Design review of the part built by this model. Coordinates are the model's own, in mm. Coordinates: 2 decimals unless noted, no trailing zeros. Loops run counter-clockwise (first coordinate to the right, second up) from the corner with the lowest first, then second, coordinate; pieces in that order, holes last. Notation, with made-up numbers: M 61.25,-2.75 L 104.25,-2.75 A14 cw 104.25,19.25 Z; hole C 11,37.5 d9. An arc over 180 degrees is marked long. Write item = value, one per line. Start each with the question number.
from build123d import *

# Parameters (mm, degrees)
ESQUISSE1_W        = 35
ESQUISSE1_H        = 23
ESQUISSE1_R        = 3.5
ESQUISSE1_R_2      = 1
ESQUISSE1_R_3      = 1.5
BOSS_EXTRU_1_DEPTH = 6


with BuildPart() as part:
    # Esquisse1 → Boss.-Extru.1 (new body)
    with BuildSketch(Plane.XY):
        Rectangle(ESQUISSE1_W, ESQUISSE1_H)
        Circle(ESQUISSE1_R, mode=Mode.SUBTRACT)
        with Locations((0, 8)):
            Circle(ESQUISSE1_R_2, mode=Mode.SUBTRACT)
        with Locations((8, 0)):
            Circle(ESQUISSE1_R_2, mode=Mode.SUBTRACT)
        with Locations((0, -8)):
            Circle(ESQUISSE1_R_2, mode=Mode.SUBTRACT)
        with Locations((-8, 0)):
            Circle(ESQUISSE1_R_2, mode=Mode.SUBTRACT)
        with Locations((-14.5, 5.75)):
            Circle(ESQUISSE1_R_3, mode=Mode.SUBTRACT)
        with Locations(Location((-14.5, -5.75, 0), (0, 0, 180))):
            Circle(ESQUISSE1_R_3, mode=Mode.SUBTRACT)
        with Locations((14.5, -5.75)):
            Circle(ESQUISSE1_R_3, mode=Mode.SUBTRACT)
        with Locations(Location((14.5, 5.75, 0), (0, 0, 180))):
            Circle(ESQUISSE1_R_3, mode=Mode.SUBTRACT)
    extrude(amount=BOSS_EXTRU_1_DEPTH)


solid = part.part
Q1. Add section D-D on z = 4.95. Give the number of separate pieces and of enclosed holes in the cut face, plus the area to 3 significant figures.
Q2. Add section C-C on y = 0. State the section outline as (x, z) points, plus the area to 3 significant figures.
Q3. Clearance check with flat-ended pins moving along their axes: P1, Ø5.5, axis at x = 0, y = 0, coming from the +Z side; P2, Ø2.5, axis at x = 0, y = -8, coming from the -Z side. State where each tip first meets the part, or that it passes through.
Q4. Add section B-B on x = 8. State the section outline as (y, z) points, plus the area to 3 significant figures.
Q5. Mouldability with a two-part tool opening along X and no side actions: class faces 1 (the face through (17.5, 0, 3)), 2 (the face through (16, 5.7, 3)), 3 (the face through (-4, 0, 0)) as released by +X, released by -X, zero draft, split by the parting line, or undercut.
Q6. Add section A-A on y = -8. State the section outline as (x, z) points, plus the area to 3 significant figures.
Q7. To check wall thickness, follow line 1 (Y direction, x = -14.5, z = 2.8); line 2 (Y direction, x = 0, z = 1.7); line 3 (X direction, y = -6, z = 1.6). State the ranges of each line that lie inside material, in increasing order. Write a range as from..to.
Values follow:
q1.separate_pieces = 1
q1.enclosed_holes = 9
q1.area = 726 mm2
q2.outline = M -17.5,0 L -9,0 L -9,6 L -17.5,6 Z; M -7,0 L -3.5,0 L -3.5,6 L -7,6 Z; M 3.5,0 L 7,0 L 7,6 L 3.5,6 Z; M 9,0 L 17.5,0 L 17.5,6 L 9,6 Z
q2.area = 144 mm2
q3.P1 = through
q3.P2 = 0
q4.outline = M -11.5,0 L -1,0 L -1,6 L -11.5,6 Z; M 1,0 L 11.5,0 L 11.5,6 L 1,6 Z
q4.area = 126 mm2
q5.face_1 = released by +X
q5.face_2 = undercut
q5.face_3 = zero draft
q6.outline = M -17.5,0 L -1,0 L -1,6 L -17.5,6 Z; M 1,0 L 17.5,0 L 17.5,6 L 1,6 Z
q6.area = 198 mm2
q7.line_1 = -11.5..-7.25, -4.25..4.25, 7.25..11.5
q7.line_2 = -11.5..-9, -7..-3.5, 3.5..7, 9..11.5
q7.line_3 = -17.5..-15.98, -13.02..13.02, 15.98..17.5
